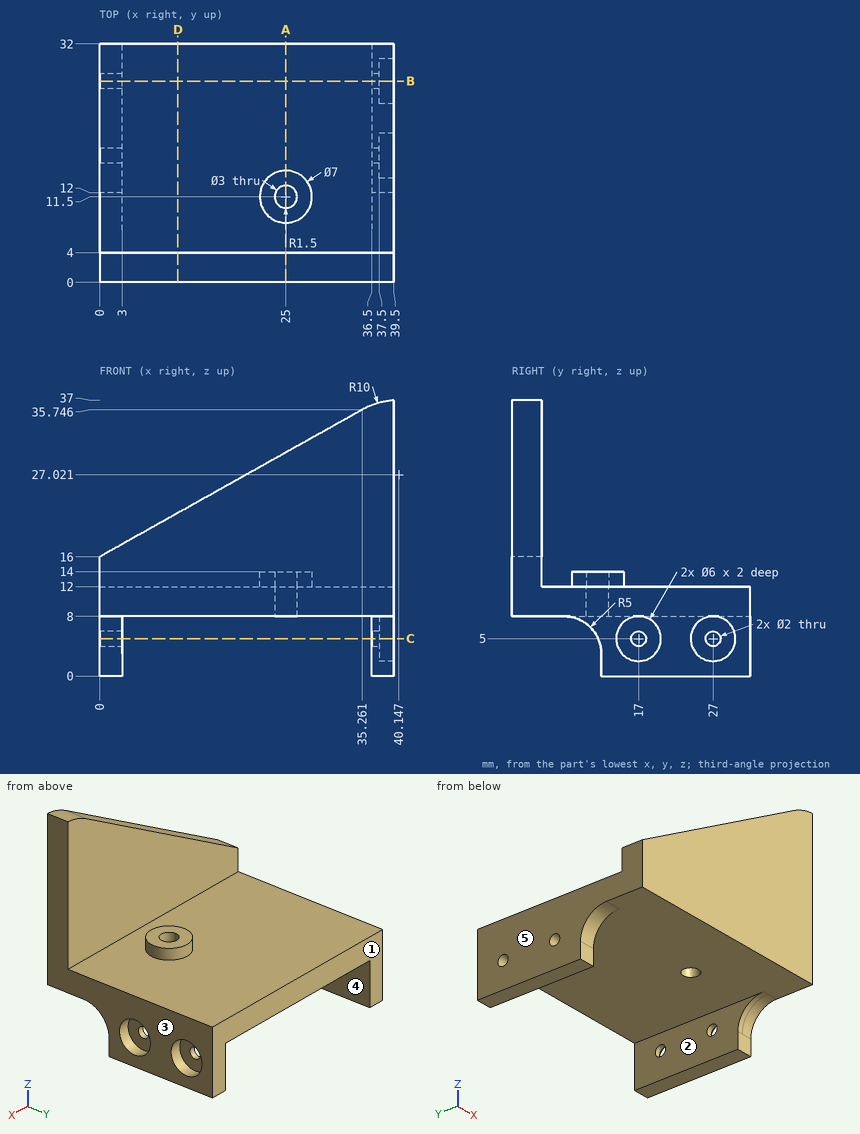
Here's the drawing with two shaded views (mm, measured from the low corner). I have some questions. A direction names the side the tool comes from. Round coordinates to 2 decimals unless told otherwise and drop trailing zeros. Loops run counter-clockwise (first coordinate to the right, second up) from the corner with the lowest first, then second, coordinate; pieces in that order, holes last. Notation, with made-up numbers: (-24, 35) - (-12, 35) arc R17 cw to (-12, 56) - close; hole circle Ø4 at (62.25, -34). An arc over 180 degrees is marked (long way). Write item = value, one per line.
1) I'm going to push flat-ended pins straight in: P1, Ø7.5, axis at x = 25, y = 13, coming from the +Z side; P2, Ø6, axis at x = 34.5, z = 31.5, coming from the +Y side; P3, Ø4, axis at x = 30.5, y = 13, coming from the +Z side; P4, Ø1.8, axis at y = 27, z = 5, coming from the -X side. Where does each tip first touch, or does it pass through?
Computed:
P1 = 14
P2 = 4
P3 = 12
P4 = through
2) On a 3-axis mill with a long thin cutter (end or side, diameter ignored), from which of +Z, -Z, +X, -X, +Y, -Y can I reach the whole of each face in a straight line? I mean the marked faces 1 and 2. Say none if no direction works.
Computed:
face_1 = +Z, -Z, +X, -X, +Y
face_2 = -Z, +Y, -Y
3) Imagine slicing it at A-A (x = 25). Please give me the cut outline in (y, z), and give its area (3 significant figures).
Computed:
outline = (0, 8) - (10, 8) - (10, 14) - (8, 14) - (8, 12) - (4, 12) - (4, 30) - (0, 30) - close; (13, 8) - (32, 8) - (32, 12) - (15, 12) - (15, 14) - (13, 14) - close
area = 196 mm2
4) Imagine slicing it at B-B (y = 27). Please give me the cut outline in (x, z), and give its area (3 significant figures).
Computed:
outline = (0, 0) - (3, 0) - (3, 4) - (0, 4) - close; (0, 6) - (3, 6) - (3, 8) - (36.5, 8) - (36.5, 6) - (37.5, 6) - (37.5, 8) - (39.5, 8) - (39.5, 12) - (0, 12) - close; (36.5, 0) - (39.5, 0) - (39.5, 2) - (37.5, 2) - (37.5, 4) - (36.5, 4) - close
area = 186 mm2
5) Imagine slicing it at C-C (z = 5). Give the number of separate pieces and of enclosed holes in the cut face.
Computed:
separate_pieces = 6
enclosed_holes = 0
6) Imagine slicing it at D-D (x = 10.5). Please give me the cut outline in (y, z).
Computed:
outline = (0, 8) - (32, 8) - (32, 12) - (4, 12) - (4, 21.88) - (0, 21.88) - close
7) If we mould it in two halves opening along X, with no side actions, what happens to the marked faces 3, 4 and 5? For each: pulls with the +X half, pulls with the -X half, needs draft (parallel to the pull), parting line crosses it, or undercut.
Computed:
face_3 = pulls with the +X half
face_4 = undercut
face_5 = pulls with the -X half
8) I need wall thicknesses on line 1 along Y through (x, z) = (37.2, 5); line 2 along Y through (x, z) = (25, 9); line 3 along Z through (x, y) = (36.7, 17). Which ranges of each line are inside material? Lowest first, please. Write a range as from..to.
Computed:
line_1 = 11.58..16, 18..26, 28..32
line_2 = 0..10, 13..32
line_3 = 0..4, 6..12
